Geometry check sheet. Reference: the model listing, model coordinates, mm. Face numbers are marked on the shaded views. Coordinates: 2 decimals unless noted, no trailing zeros. Write each loop counter-clockwise with the first axis right and the second up, starting at its lowest first coordinate (ties: lowest second). Pieces come first, ordered by that corner, then holes. Notation, with made-up numbers: (12.5, -11) -> (46.5, -11) arc R25 ccw to (46.5, 21) -> close; hole circle Ø8 at (30.25, 80.5). An arc over 180 degrees is marked (long way). One line per question, with ' | ' between items.
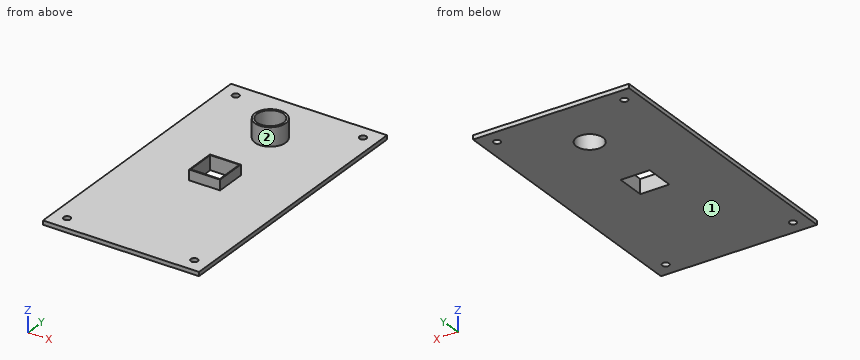
Autodesk Fusion 360 part; units mm, degrees
sketch "Sketch1" plane through (0, 0, 0) normal (0, 0, 1) x (1, 0, 0)
  line L0 (38, 68) -> (-38, 68)
  line L1 (-38, 68) -> (-38, -68)
  line L2 (-38, -68) -> (38, -68)
  line L3 (38, -68) -> (38, 68)
  line L4 (38, 68) -> (-38, -68) construction
  line L5 (-38, 68) -> (38, -68) construction
  line L6 (7.1, 7.1) -> (-7.1, 7.1)
  line L7 (-7.1, 7.1) -> (-7.1, -7.1)
  line L8 (-7.1, -7.1) -> (7.1, -7.1)
  line L9 (7.1, -7.1) -> (7.1, 7.1)
  line L10 (7.1, 7.1) -> (-7.1, -7.1) construction
  line L11 (-7.1, 7.1) -> (7.1, -7.1) construction
  circle A0 centre (0, 40) radius 6.5
  circle A1 centre (0, 40) radius 7.5
  line L12 (-38, 68) -> (-31, 68)
  line L13 (-31, 68) -> (-31, 61)
  line L14 (-31, 61) -> (-38, 61)
  line L15 (-38, 61) -> (-38, 68)
  circle A2 centre (-31, 61) radius 1.7
  line L16 (38, 68) -> (31, 68)
  line L17 (31, 68) -> (31, 61)
  line L18 (31, 61) -> (38, 61)
  line L19 (38, 61) -> (38, 68)
  circle A3 centre (31, 61) radius 1.7
  circle A4 centre (-31, -61) radius 1.7
  circle A5 centre (31, -61) radius 1.7
  line L20 (7.5, 7.5) -> (-7.5, 7.5)
  line L21 (-7.5, 7.5) -> (-7.5, -7.5)
  line L22 (-7.5, -7.5) -> (7.5, -7.5)
  line L23 (7.5, -7.5) -> (7.5, 7.5)
  line L24 (7.5, 7.5) -> (-7.5, -7.5) construction
  line L25 (-7.5, 7.5) -> (7.5, -7.5) construction
  dimension "d1" = 76
  dimension "d2" = 136
  dimension "d3" = 14.2
  dimension "d4" = 14.2
  dimension "d5" = 13
  dimension "d6" = 1
  dimension "d7" = 7
  dimension "d8" = 7
  dimension "d9" = 3.4
  dimension "d10" = 7
  dimension "d11" = 7
  dimension "d14" = 62
  dimension "d15" = -122
  dimension "d16" = 15
  dimension "d17" = 15
extrude "Extrude1" add sketch "Sketch1" along normal blind 2 contours L0 L3 L16 L17 L18 L19 A3 | L0 L1 L2 L3 L13 L14 A2 L17 L18 A3 | L0 L1 L12 L13 L14 L15 A2
extrude "Extrude2" add sketch "Sketch1" along normal blind 11 contours A1
extrude "Extrude3" add sketch "Sketch1" along normal blind 7 contours L20 L21 L22 L23
1. Cross-section at B-B on x = 0. Record the boundary of the cut face in (y, z), and give its area (3 significant figures).
Worked answers:
outline: (-68, 0) -> (-7.1, 0) -> (-7.1, 7) -> (-7.5, 7) -> (-7.5, 2) -> (-68, 2) -> close; (7.1, 0) -> (33.5, 0) -> (33.5, 11) -> (32.5, 11) -> (32.5, 2) -> (7.5, 2) -> (7.5, 7) -> (7.1, 7) -> close; (46.5, 0) -> (68, 0) -> (68, 2) -> (47.5, 2) -> (47.5, 11) -> (46.5, 11) -> close | area: 240 mm²
2. Cross-section at A-A on z = 5. Record the boundary of the cut face in (x, y).
Worked answers:
outline: (-7.5, -7.5) -> (7.5, -7.5) -> (7.5, 7.5) -> (-7.5, 7.5) -> close; circle Ø15 at (0, 40); hole (-7.1, -7.1) -> (7.1, -7.1) -> (7.1, 7.1) -> (-7.1, 7.1) -> close; hole circle Ø13 at (0, 40)
3. Mould release check, pull along Y, two halves, no side actions. Record for the marked faces 1 and 2: released by +Y, released by -Y, zero draft, split by the parting line, or undercut.
Worked answers:
face 1: zero draft | face 2: undercut
4. Go/stop test with flat-tipped pins: P1, Ø4.5, axis at x = -31, y = -61, coming from the +Z side; P2, Ø2, axis at x = 31, y = 61, coming from the +Z side; P3, Ø1.5, axis at y = 0.5, z = 5, coming from the +X side. Record where each tip stops, or that it passes through.
Worked answers:
P1: z = 2 | P2: through | P3: x = 7.5
5. Material ranges on line 1 (Y direction, x = -31, z = 1.55); line 2 (X direction, y = 3, z = 6.5); line 3 (Z direction, x = 4.5, y = 17), recorded low to high. Write a range as from..to.
Worked answers:
line 1: -68..-62.7, -59.3..59.3, 62.7..68 | line 2: -7.5..-7.1, 7.1..7.5 | line 3: 0..2
6. Cross-section at C-C on y = 1. Record the boundary of the cut face in (x, z), and give its area (3 significant figures).
Worked answers:
outline: (-38, 0) -> (-7.1, 0) -> (-7.1, 7) -> (-7.5, 7) -> (-7.5, 2) -> (-38, 2) -> close; (7.1, 0) -> (38, 0) -> (38, 2) -> (7.5, 2) -> (7.5, 7) -> (7.1, 7) -> close | area: 128 mm²
7. Cross-section at D-D on x = 31. Record the boundary of the cut face in (y, z), and give its area (3 significant figures).
Worked answers:
outline: (-68, 0) -> (-62.7, 0) -> (-62.7, 2) -> (-68, 2) -> close; (-59.3, 0) -> (59.3, 0) -> (59.3, 2) -> (-59.3, 2) -> close; (62.7, 0) -> (68, 0) -> (68, 2) -> (62.7, 2) -> close | area: 258 mm²
